Input: part model. Units: mm. Frame: model coordinates. Face numbers are marked on the shaded views. A direction names the side the tool comes from. Round coordinates to 2 decimals unless told otherwise and drop trailing zeros. Loops run counter-clockwise (first coordinate to the right, second up) from the corner with the lowest first, then second, coordinate; pieces in that order, holes last. Notation, with made-up numbers: (-38, -36) -> (-4, -36) arc R29 cw to (-4, 2) -> close; hole circle Ø8 at (52, 64). An arc over 180 degrees is marked (long way). Answer as a JSON object with one key per item and string values. Group by question number.
Item 1: Draft query along X for the marked faces 1, 2 and 3. Return one class per face: released by +X, released by -X, zero draft, split by the parting line, or undercut.
Item 2: Pin query (flat end, axial travel): pin 1 (2 mm diameter, centred on x = -3.5, z = -34, fed in from +Y); pin 2 (2 mm diameter, centred on x = -6, z = 20, fed in from -Y); pin 3 (2 mm diameter, centred on y = 0, z = 0, fed in from +X); pin 4 (3 mm diameter, centred on y = -12.41, z = 16.38, fed in from -X). Return the tip coordinate at first contact, or that it passes through.
Item 3: Section query A-A on z = 27. Return loops of the section in (x, y).
Item 4: Set-up query: the marked faces 4, 5 and 6. Return all of +Z, -Z, +X, -X, +Y, -Y with unobstructed straight access to the full face (end or side cutting, diameter ignored); none if empty.
Item 5: Material intervals for line 1 (X direction, y = 31.5, z = -19); line 2 (Z direction, x = 11, y = 5); line 3 (Y direction, x = -8, z = 5), sorted ascending. Write a range as [from, to].
Item 6: Section query B-B on y = -33. Return loops of the section in (x, z).
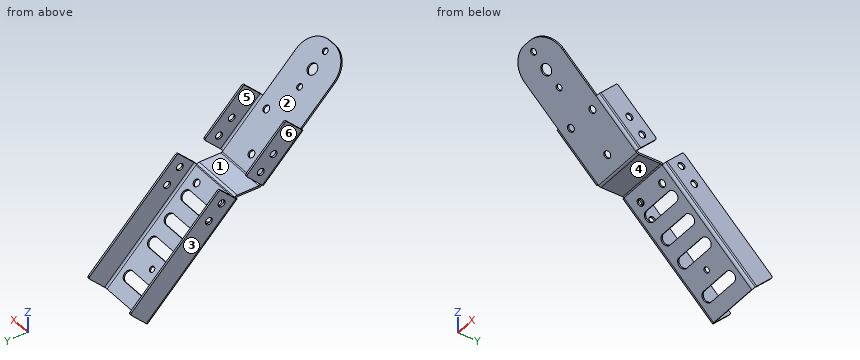
from build123d import *

# Parameters (mm, degrees)
BASE_FLANGE1_DEPTH     = 1
SKETCHED_START         = -30
SKETCHED_BEND5_DEPTH   = 60
SKETCHED_BEND5_2_DEPTH = 15
SKETCHED_START_2       = 15
SKETCHED_BEND5_3_DEPTH = 15
SKETCHED_BEND5_4_DEPTH = 60
SKETCHED_START_3       = -15
SKETCHED_BEND5_5_DEPTH = 30
SKETCHED_BEND6_DEPTH   = 60
SKETCHED_BEND6_2_DEPTH = 15
SKETCHED_BEND6_3_DEPTH = 15
SKETCHED_BEND6_4_DEPTH = 30
SKETCHED_BEND6_5_DEPTH = 60
SKETCHED_START_4       = -36.356310605
SKETCHED_BEND7_DEPTH   = 31
SKETCHED_BEND7_2_DEPTH = 31
SKETCHED_START_5       = 5.890889039
SKETCHED_BEND8_DEPTH   = 70
SKETCHED_BEND8_2_DEPTH = 70
CUT_EXTRUDE1_DEPTH     = 10
F_6_CLEARANCE_HOLE4_D  = 3.7973
F_6_CLEARANCE_HOLE2_D  = 3.7973
FILLET1_R              = 1
F_4_CLEARANCE_HOLE1_D  = 3.2639
F_6_0MM_DOWEL_HOLE1_D  = 6
F_3_0MM_DOWEL_HOLE1_D  = 3
FILLET2_R              = 13


# Read off the part's stored shape, not the designer's step: Sketched Bend5, Sketched Bend6, Sketched Bend7, Sketched Bend8
# Sheet-metal steps are written as plain solids
with BuildPart() as part:
    # Sketch1 → Base-Flange1 (new body)
    with BuildSketch(Plane.XY):
        Polygon((-30, -38.5), (-15, -38.5), (-15, -77.5), (15, -77.5), (15, -38.5), (30, -38.5), (30, -7.5), (15, -7.5), (15, 7.5), (30, 7.5), (30, 77.5), (15, 77.5), (-15, 77.5), (-30, 77.5), (-30, 7.5), (-15, 7.5), (-15, -7.5), (-30, -7.5), align=None)
    extrude(amount=-BASE_FLANGE1_DEPTH)

    # Sketched Bend5 outline → Sketched Bend5 (cut)
    with BuildSketch(Plane.YZ.offset(SKETCHED_START)):
        with BuildLine():
            Line((7.714213562, -0.585786438), (8.128427124, -1))
            Line((8.128427124, -1), (77.5, -1))
            Line((77.5, -1), (77.5, 0))
            Line((77.5, 0), (6.3, 0))
            ThreePointArc((6.3, 0), (7.065366865, -0.152240935), (7.714213562, -0.585786438))
        make_face()
    extrude(amount=SKETCHED_BEND5_DEPTH, mode=Mode.SUBTRACT)

    # Sketched Bend5 2 outline → Sketched Bend5 2 (cut)
    with BuildSketch(Plane.YZ.offset(SKETCHED_START)):
        with BuildLine():
            Line((7.729701149, -0.601274024), (7.714213562, -0.585786438))
            ThreePointArc((7.714213562, -0.585786438), (7.610403483, -0.48909209), (7.5, -0.4))
            Line((7.5, -0.4), (7.5, -0.830975173))
            Line((7.5, -0.830975173), (7.729701149, -0.601274024))
        make_face()
    extrude(amount=SKETCHED_BEND5_2_DEPTH, mode=Mode.SUBTRACT)

    # Sketched Bend5 3 outline → Sketched Bend5 3 (cut)
    with BuildSketch(Plane.YZ.offset(SKETCHED_START_2)):
        with BuildLine():
            Line((7.729701149, -0.601274024), (7.714213562, -0.585786438))
            ThreePointArc((7.714213562, -0.585786438), (7.610403483, -0.48909209), (7.5, -0.4))
            Line((7.5, -0.4), (7.5, -0.830975173))
            Line((7.5, -0.830975173), (7.729701149, -0.601274024))
        make_face()
    extrude(amount=SKETCHED_BEND5_3_DEPTH, mode=Mode.SUBTRACT)

    # Sketched Bend5 4 outline → Sketched Bend5 4 (add)
    with BuildSketch(Plane.YZ.offset(SKETCHED_START)):
        Polygon((57.227175832, -50.098748707), (8.128427124, -1), (7.5, -1), (7.5, -0.830975173), (7.022594368, -1.308380805), (56.520069051, -50.805855488), align=None)
    extrude(amount=SKETCHED_BEND5_4_DEPTH)

    # Sketched Bend5 5 outline → Sketched Bend5 5 (add)
    with BuildSketch(Plane.YZ.offset(SKETCHED_START_3)):
        with BuildLine():
            Line((7.022594368, -1.308380805), (7.330975173, -1))
            Line((7.330975173, -1), (6.3, -1))
            ThreePointArc((6.3, -1), (6.682683432, -1.076120467), (7.007106781, -1.292893219))
            Line((7.007106781, -1.292893219), (7.022594368, -1.308380805))
        make_face()
    extrude(amount=SKETCHED_BEND5_5_DEPTH)

    # Sketched Bend6 outline → Sketched Bend6 (cut)
    with BuildSketch(Plane.YZ.offset(SKETCHED_START)):
        with BuildLine():
            ThreePointArc((-5.710951377, -1), (-6.476318242, -0.847759065), (-7.12516494, -0.414213562))
            Line((-7.12516494, -0.414213562), (-7.539378502, 0))
            Line((-7.539378502, 0), (-77.5, 0))
            Line((-77.5, 0), (-77.5, -1))
            Line((-77.5, -1), (-5.710951377, -1))
        make_face()
    extrude(amount=SKETCHED_BEND6_DEPTH, mode=Mode.SUBTRACT)

    # Sketched Bend6 2 outline → Sketched Bend6 2 (cut)
    with BuildSketch(Plane.YZ.offset(SKETCHED_START)):
        Polygon((-7.539378502, 0), (-7.5, -0.039378502), (-7.5, 0), align=None)
    extrude(amount=SKETCHED_BEND6_2_DEPTH, mode=Mode.SUBTRACT)

    # Sketched Bend6 3 outline → Sketched Bend6 3 (cut)
    with BuildSketch(Plane.YZ.offset(SKETCHED_START_2)):
        Polygon((-7.539378502, 0), (-7.5, -0.039378502), (-7.5, 0), align=None)
    extrude(amount=SKETCHED_BEND6_3_DEPTH, mode=Mode.SUBTRACT)

    # Sketched Bend6 4 outline → Sketched Bend6 4 (add)
    with BuildSketch(Plane.YZ.offset(SKETCHED_START_3)):
        with BuildLine():
            Line((-7.539378502, 0), (-5.710951377, 0))
            ThreePointArc((-5.710951377, 0), (-6.09363481, 0.076120467), (-6.418058159, 0.292893219))
            Line((-6.418058159, 0.292893219), (-56.347540704, 50.222375764))
            Line((-56.347540704, 50.222375764), (-57.054647485, 49.515268983))
            Line((-57.054647485, 49.515268983), (-7.539378502, 0))
        make_face()
    extrude(amount=SKETCHED_BEND6_4_DEPTH)

    # Sketched Bend6 5 outline → Sketched Bend6 5 (add)
    with BuildSketch(Plane.YZ.offset(SKETCHED_START)):
        Polygon((-29.477483019, 21.938104517), (-7.557172802, 0.0177943), (-6.850066021, 0.724901081), (-28.770376238, 22.645211298), align=None)
    extrude(amount=SKETCHED_BEND6_5_DEPTH)

    # Sketched Bend7 outline → Sketched Bend7 (cut)
    with BuildSketch(Plane(origin=(0, 0, 0), x_dir=(1, 0, 0), z_dir=(0, 0.707106781186546, -0.707106781186549)).offset(SKETCHED_START_4)):
        with BuildLine():
            ThreePointArc((-16.732050807, 4.331145665), (-16, 5.063196472), (-15, 5.331145665))
            Line((-15, 5.331145665), (-30, 5.331145665))
            Line((-30, 5.331145665), (-30, 4.331145665))
            Line((-30, 4.331145665), (-16.732050807, 4.331145665))
        make_face()
        with BuildLine():
            Line((30, 5.331145665), (15, 5.331145665))
            ThreePointArc((15, 5.331145665), (16, 5.063196472), (16.732050807, 4.331145665))
            Line((16.732050807, 4.331145665), (30, 4.331145665))
            Line((30, 4.331145665), (30, 5.331145665))
        make_face()
    extrude(amount=SKETCHED_BEND7_DEPTH, mode=Mode.SUBTRACT)

    # Sketched Bend7 2 outline → Sketched Bend7 2 (add)
    with BuildSketch(Plane(origin=(0, 0, 0), x_dir=(1, 0, 0), z_dir=(0, 0.707106781186546, -0.707106781186549)).offset(SKETCHED_START_4)):
        with BuildLine():
            Line((-15, 4.331145665), (-16.732050807, 4.331145665))
            ThreePointArc((-16.732050807, 4.331145665), (-16.931851652, 3.848783755), (-17, 3.331145665))
            Line((-17, 3.331145665), (-17, -9.312659845))
            Line((-17, -9.312659845), (-16, -9.312659845))
            Line((-16, -9.312659845), (-16, 3.331145665))
            ThreePointArc((-16, 3.331145665), (-15.707106781, 4.038252446), (-15, 4.331145665))
        make_face()
        with BuildLine():
            ThreePointArc((17, 3.331145665), (16.931851652, 3.848783755), (16.732050807, 4.331145665))
            Line((16.732050807, 4.331145665), (15, 4.331145665))
            ThreePointArc((15, 4.331145665), (15.707106781, 4.038252446), (16, 3.331145665))
            Line((16, 3.331145665), (16, -9.312659845))
            Line((16, -9.312659845), (17, -9.312659845))
            Line((17, -9.312659845), (17, 3.331145665))
        make_face()
    extrude(amount=SKETCHED_BEND7_2_DEPTH)

    # Sketched Bend8 outline → Sketched Bend8 (cut)
    with BuildSketch(Plane(origin=(0, 0, 0), x_dir=(1, 0, 0), z_dir=(0, 0.707106781186546, -0.707106781186549)).offset(SKETCHED_START_5)):
        with BuildLine():
            Line((-30, -5.040559159), (-16.732050807, -5.040559159))
            ThreePointArc((-16.732050807, -5.040559159), (-16, -4.308508352), (-15, -4.040559159))
            Line((-15, -4.040559159), (-30, -4.040559159))
            Line((-30, -4.040559159), (-30, -5.040559159))
        make_face()
        with BuildLine():
            Line((30, -4.040559159), (15, -4.040559159))
            ThreePointArc((15, -4.040559159), (16, -4.308508352), (16.732050807, -5.040559159))
            Line((16.732050807, -5.040559159), (30, -5.040559159))
            Line((30, -5.040559159), (30, -4.040559159))
        make_face()
    extrude(amount=SKETCHED_BEND8_DEPTH, mode=Mode.SUBTRACT)

    # Sketched Bend8 2 outline → Sketched Bend8 2 (add)
    with BuildSketch(Plane(origin=(0, 0, 0), x_dir=(1, 0, 0), z_dir=(0, 0.707106781186546, -0.707106781186549)).offset(SKETCHED_START_5)):
        with BuildLine():
            ThreePointArc((-16.732050807, -5.040559159), (-16.931851652, -5.522921069), (-17, -6.040559159))
            Line((-17, -6.040559159), (-17, -18.684364669))
            Line((-17, -18.684364669), (-16, -18.684364669))
            Line((-16, -18.684364669), (-16, -6.040559159))
            ThreePointArc((-16, -6.040559159), (-15.707106781, -5.333452378), (-15, -5.040559159))
            Line((-15, -5.040559159), (-16.732050807, -5.040559159))
        make_face()
        with BuildLine():
            Line((16.732050807, -5.040559159), (15, -5.040559159))
            ThreePointArc((15, -5.040559159), (15.707106781, -5.333452378), (16, -6.040559159))
            Line((16, -6.040559159), (16, -18.684364669))
            Line((16, -18.684364669), (17, -18.684364669))
            Line((17, -18.684364669), (17, -6.040559159))
            ThreePointArc((17, -6.040559159), (16.931851652, -5.522921069), (16.732050807, -5.040559159))
        make_face()
    extrude(amount=SKETCHED_BEND8_2_DEPTH)

    # Sketch36 → Cut-Extrude1 (cut)
    with BuildSketch(Plane(origin=(0, 3.564213562, 3.564213562), x_dir=(1, 0, 0), z_dir=(0, 0.7071067811865487, 0.7071067811865465))):
        with BuildLine():
            Line((-9, 23), (9, 23))
            ThreePointArc((9, 23), (12, 20), (9, 17))
            Line((9, 17), (-9, 17))
            ThreePointArc((-9, 17), (-12, 20), (-9, 23))
        make_face()
        with BuildLine():
            Line((-9, 36), (9, 36))
            ThreePointArc((9, 36), (12, 33), (9, 30))
            Line((9, 30), (-9, 30))
            ThreePointArc((-9, 30), (-12, 33), (-9, 36))
        make_face()
        with BuildLine():
            Line((-9, 49), (9, 49))
            ThreePointArc((9, 49), (12, 46), (9, 43))
            Line((9, 43), (-9, 43))
            ThreePointArc((-9, 43), (-12, 46), (-9, 49))
        make_face()
        with BuildLine():
            Line((-9, 68), (9, 68))
            ThreePointArc((9, 68), (12, 65), (9, 62))
            Line((9, 62), (-9, 62))
            ThreePointArc((-9, 62), (-12, 65), (-9, 68))
        make_face()
    extrude(amount=-CUT_EXTRUDE1_DEPTH, mode=Mode.SUBTRACT)

    # #6 Clearance Hole4 (through all)
    with Locations(Plane(origin=(0, 3.564213562, 3.564213562), x_dir=(1, 0, 0), z_dir=(0, 0.7071067811865487, 0.7071067811865465))):
        with Locations((-8.5, 12.368986284), (8.5, 12.368986284), (0, -12.745359227), (-8.5, -32.745359227), (8.5, -32.745359227)):
            Hole(F_6_CLEARANCE_HOLE4_D / 2)

    # #6 Clearance Hole2 (through all)
    with Locations(Plane(origin=(17, 0, 0), x_dir=(0, 0, -1), z_dir=(1, 0, 0))):
        with Locations((-9.311868306, -5.334166607), (-16.382936118, -12.405234419), (-0.914625389, 16.316668374), (6.156442422, 23.387736186)):
            Hole(F_6_CLEARANCE_HOLE2_D / 2)

    # Fillet1
    fillet1_edges = [part.edges().sort_by_distance(p)[0] for p in [
        (-16.5, -19.12274884, 32.292838695),
        (-16.5, 2.797561376, 10.372528478),
        (16.5, 2.797561376, 10.372528478),
        (16.5, -19.12274884, 32.292838695),
        (-16.5, 17.377328546, 9.046353373),
        (-16.5, 66.874803229, -40.45112131),
        (16.5, 66.874803229, -40.45112131),
        (16.5, 17.377328546, 9.046353373),
    ]]
    fillet(fillet1_edges, radius=FILLET1_R)

    # #4 Clearance Hole1 (through all)
    with Locations(Plane(origin=(0, -3.06258247, -3.06258247), x_dir=(1, 0, 0), z_dir=(0, 0.7071067811865487, 0.7071067811865465))):
        with Locations((0, -70.356310605), (0, -50.356310605)):
            Hole(F_4_CLEARANCE_HOLE1_D / 2)

    # Ø6.0mm Dowel Hole1 (through all)
    with Locations(Plane(origin=(0, -3.06258247, -3.06258247), x_dir=(1, 0, 0), z_dir=(0, 0.7071067811865487, 0.7071067811865465))):
        with Locations((0, -60.356310605)):
            Hole(F_6_0MM_DOWEL_HOLE1_D / 2)

    # Ø3.0mm Dowel Hole1 (through all)
    with Locations(Plane(origin=(0, 3.564213562, 3.564213562), x_dir=(1, 0, 0), z_dir=(0, 0.7071067811865487, 0.7071067811865465))):
        with Locations((0, 55.530889039)):
            Hole(F_3_0MM_DOWEL_HOLE1_D / 2)

    # Fillet2
    fillet2_edges = [part.edges().sort_by_distance(p)[0] for p in [
        (-15, -56.701094094, 49.868822373),
        (15, -56.701094094, 49.868822373),
    ]]
    fillet(fillet2_edges, radius=FILLET2_R)


solid = part.part
Solved:
{
 "1": {"face 1": "zero draft", "face 2": "undercut", "face 3": "released by -X"},
 "2": {"pin 1": "y = 42.13", "pin 2": "y = -28.54", "pin 3": "x = 15", "pin 4": "through"},
 "3": {"outline": "(-17, -24.42) -> (-16, -24.42) -> (-16, -13.83) -> (-17, -13.83) -> close; (-15, -34.54) -> (15, -34.54) -> (15, -33.13) -> (-15, -33.13) -> close; (16, -24.42) -> (17, -24.42) -> (17, -13.83) -> (16, -13.83) -> close"},
 "4": {"face 4": "-Z, +X, -X, -Y", "face 5": "+Z, +Y", "face 6": "+Z, -Z, -X, +Y, -Y"},
 "5": {"line 1": "[-17, -16], [16, 17]", "line 2": "[-1, 0]", "line 3": "[-12.54, -11.13]"},
 "6": {"outline": "(-15, 25.46) -> (15, 25.46) -> (15, 26.87) -> (-15, 26.87) -> close"}
}
